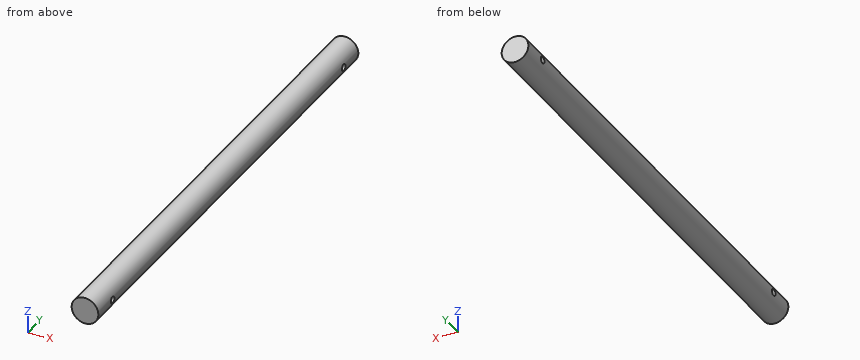
```python
from build123d import *

# Parameters (mm, degrees)
SKETCH1_R               = 25.4
BOSS_EXTRUDE1_DEPTH     = 914.4
SKETCH2_R               = 6.35
CUT_EXTRUDE3_DEPTH      = 26.4
CUT_EXTRUDE3_DEPTH_BACK = 26.4


with BuildPart() as part:
    # Sketch1 → Boss-Extrude1 (new body)
    with BuildSketch(Plane(origin=(0, 0, 0), x_dir=(1, 0, 0), z_dir=(0, 1, 0))):
        Circle(SKETCH1_R)
    extrude(amount=BOSS_EXTRUDE1_DEPTH)

    # Sketch2 → Cut-Extrude3 (cut, two sides)
    with BuildSketch(Plane(origin=(0, 0, 0), x_dir=(0, 0, -1), z_dir=(1, 0, 0))) as cut_extrude3_sk:
        with Locations((0, 863.6)):
            Circle(SKETCH2_R)
        with Locations((0, 50.8)):
            Circle(SKETCH2_R)
    extrude(amount=CUT_EXTRUDE3_DEPTH, mode=Mode.SUBTRACT)
    extrude(cut_extrude3_sk.sketch, amount=-CUT_EXTRUDE3_DEPTH_BACK, mode=Mode.SUBTRACT)


solid = part.part
```
For this review, take the finished solid that the model builds, in its own axes (mm). Give positions to 0.01 mm unless a question says otherwise; leave off trailing zeros. Order: outer loops, then holes, each group sorted by start corner. A loop starts at its lowest first (then second) coordinate and runs counter-clockwise, first axis right, second up.
1) Take a section at A-A (x = -11). Give the boundary of the cut face in (y, z).
2) Wall thickness on line 1 (Y direction, x = 19.5, z = 1.5); line 2 (Y direction, x = 16.5, z = 0); line 3 (Z direction, x = -2, y = 329): over which ranges is each line inside the solid? List them lowest first.
3) Take a section at B-B (y = 237.5). Give the boundary of the cut face in (x, z), then the cut area to 3 significant figures.
4) Take a section at C-C (z = 16). Give the boundary of the cut face in (x, y).
5) Insertion check: pin 1 (3 mm diameter, centred on y = 644, z = -11.5, fed in from +X); pin 2 (6 mm diameter, centred on x = -6.5, y = 117, fed in from -Z); pin 3 (8 mm diameter, centred on x = -19.5, y = 201.5, fed in from -Z); pin 4 (7.5 mm diameter, centred on y = 50.8, z = 0, fed in from -X). Each pin has a flat end and moves straight along its axis. Give the tip position at first contact, or say it passes through.
Derived:
1. outline: (0, -22.89) - (914.4, -22.89) - (914.4, 22.89) - (0, 22.89) - close; hole circle Ø12.7 at (50.8, 0); hole circle Ø12.7 at (863.6, 0)
2. line 1: y = 0 to 44.63, 56.97 to 857.43, 869.77 to 914.4
2. line 2: y = 0 to 44.45, 57.15 to 857.25, 869.95 to 914.4
2. line 3: z = -25.32 to 25.32
3. outline: circle Ø50.8 at (0, 0)
3. area: 2,030 mm2
4. outline: (-19.73, 0) - (19.73, 0) - (19.73, 914.4) - (-19.73, 914.4) - close
5. pin 1: stops at x = 23.35
5. pin 2: stops at z = -25.16
5. pin 3: stops at z = -20.12
5. pin 4: passes through
